from build123d import *

# Parameters (mm, degrees)
EXTRUDE_1_DEPTH = 0.7
EXTRUDE_3_DEPTH = 2.7


with BuildPart() as part:
    # Sketch 1 → Extrude 1 (new body)
    with BuildSketch(Plane(origin=(0, 0, 0), x_dir=(1, 0, 0), z_dir=(0, 1, 0))):
        with BuildLine():
            Line((-2.916666667, 5.483035714), (0.383333333, 5.483035714))
            ThreePointArc((0.383333333, 5.483035714), (1.090440115, 5.190142495), (1.383333333, 4.483035714))
            Line((1.383333333, 4.483035714), (1.383333333, -1.016964286))
            ThreePointArc((1.383333333, -1.016964286), (1.090440115, -1.724071067), (0.383333333, -2.016964286))
            Line((0.383333333, -2.016964286), (-2.916666667, -2.016964286))
            ThreePointArc((-2.916666667, -2.016964286), (-3.623773448, -1.724071067), (-3.916666667, -1.016964286))
            Line((-3.916666667, -1.016964286), (-3.916666667, 4.483035714))
            ThreePointArc((-3.916666667, 4.483035714), (-3.623773448, 5.190142495), (-2.916666667, 5.483035714))
        make_face()
        with BuildLine():
            ThreePointArc((-1.716666667, 4.133035714), (-2.423773448, 3.840142495), (-2.716666667, 3.133035714))
            Line((-2.716666667, 3.133035714), (-2.716666667, 0.333035714))
            ThreePointArc((-2.716666667, 0.333035714), (-2.423773448, -0.374071067), (-1.716666667, -0.666964286))
            Line((-1.716666667, -0.666964286), (-0.816666667, -0.666964286))
            ThreePointArc((-0.816666667, -0.666964286), (-0.109559885, -0.374071067), (0.183333333, 0.333035714))
            Line((0.183333333, 0.333035714), (0.183333333, 3.133035714))
            ThreePointArc((0.183333333, 3.133035714), (-0.109559885, 3.840142495), (-0.816666667, 4.133035714))
            Line((-0.816666667, 4.133035714), (-1.716666667, 4.133035714))
        make_face(mode=Mode.SUBTRACT)
    extrude(amount=EXTRUDE_1_DEPTH)

    # Sketch 1_6 → Extrude 3 (add)
    with BuildSketch(Plane(origin=(0, 0, 0), x_dir=(1, 0, 0), z_dir=(0, 1, 0))):
        with BuildLine():
            Line((-1.716666667, 4.133035714), (-0.816666667, 4.133035714))
            ThreePointArc((-0.816666667, 4.133035714), (-0.109559885, 3.840142495), (0.183333333, 3.133035714))
            Line((0.183333333, 3.133035714), (0.183333333, 0.333035714))
            ThreePointArc((0.183333333, 0.333035714), (-0.109559885, -0.374071067), (-0.816666667, -0.666964286))
            Line((-0.816666667, -0.666964286), (-1.716666667, -0.666964286))
            ThreePointArc((-1.716666667, -0.666964286), (-2.423773448, -0.374071067), (-2.716666667, 0.333035714))
            Line((-2.716666667, 0.333035714), (-2.716666667, 3.133035714))
            ThreePointArc((-2.716666667, 3.133035714), (-2.423773448, 3.840142495), (-1.716666667, 4.133035714))
        make_face()
    extrude(amount=EXTRUDE_3_DEPTH)


solid = part.part
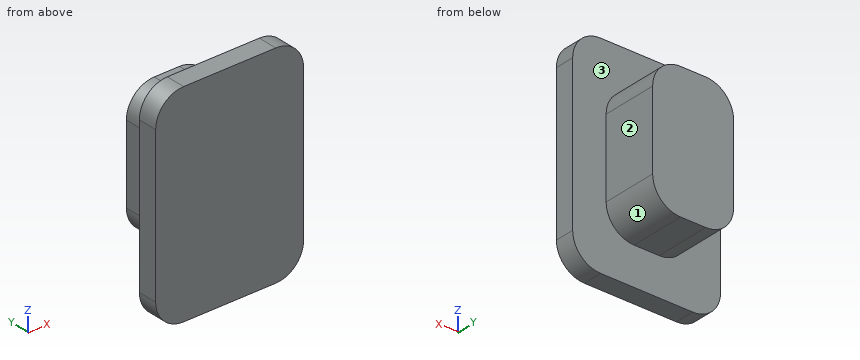
Verification items for the finished model (mm, model axes). Face numbers are marked on the shaded views. A direction names the side the tool comes from. Give positions to 0.01 mm unless a question says otherwise; leave off trailing zeros. Write each loop counter-clockwise with the first axis right and the second up, starting at its lowest first coordinate (ties: lowest second). Pieces come first, ordered by that corner, then holes. Notation, with made-up numbers: (85, 49.5) -> (114, 49.5) arc R11 ccw to (114, 53.5) -> close; hole circle Ø9 at (61.25, 59). An arc over 180 degrees is marked (long way). Use CSV: the item, a comma, the result in double quotes.
(1) Sectioned sample at D-D (z = -4.25). Record the cut outline in (x, y), plus the area to 3 significant figures.
Derived:
outline,"(-3.92, 0) -> (1.38, 0) -> (1.38, 0.7) -> (-3.92, 0.7) -> close"
area,"3.71 mm^2"
(2) Set-up check for the marked faces 1, 2 and 3: record each of +Z, -Z, +X, -X, +Y, -Y from which the full face is reachable in a straight line by a thin tool's end or side.
Derived:
face 1,"-Z, +X, +Y"
face 2,"+Z, -Z, +X, +Y"
face 3,"+Y"
(3) Material ranges on L1, parallel to Y at x = -2.4, z = -4; L2, parallel to X at y = 2.65, z = -2.75; L3, parallel to Z at x = -1.4, y = 1.55, recorded low to high.
Derived:
L1,"y = 0 to 0.7"
L2,"x = -2.72 to 0.18"
L3,"z = -4.13 to 0.67"
(4) Go/stop test with a flat-tipped pin: pin 1 (0.7 mm diameter, centred on x = -1.5, y = 1.5, fed in from -Z). Record where the tip stops, or that it passes through.
Derived:
pin 1,"stops at z = -4.13"
(5) Sectioned sample at B-B (y = 0.55). Record the cut outline in (x, z), plus the area to 3 significant figures.
Derived:
outline,"(-3.92, -4.48) arc R1 ccw to (-2.92, -5.48) -> (0.38, -5.48) arc R1 ccw to (1.38, -4.48) -> (1.38, 1.02) arc R1 ccw to (0.38, 2.02) -> (-2.92, 2.02) arc R1 ccw to (-3.92, 1.02) -> close"
area,"38.9 mm^2"
(6) Sectioned sample at C-C (x = 0.3). Record the cut outline in (y, z).
Derived:
outline,"(0, -5.48) -> (0.7, -5.48) -> (0.7, 2.02) -> (0, 2.02) -> close"
(7) Sectioned sample at A-A (z = -2). Record the cut outline in (x, y), plus the area to 3 significant figures.
Derived:
outline,"(-3.92, 0) -> (1.38, 0) -> (1.38, 0.7) -> (0.18, 0.7) -> (0.18, 2.7) -> (-2.72, 2.7) -> (-2.72, 0.7) -> (-3.92, 0.7) -> close"
area,"9.51 mm^2"
